from build123d import *

# Parameters (mm, degrees)
CROQUIS1_R              = 7.5
SALIENTE_EXTRUIR1_DEPTH = 10


with BuildPart() as part:
    # Croquis1 → Saliente-Extruir1 (new body)
    with BuildSketch(Plane(origin=(0, 0, 0), x_dir=(1, 0, 0), z_dir=(0, 1, 0))):
        with BuildLine():
            Line((-35, 35), (35, 35))
            Line((35, 35), (35, -25))
            ThreePointArc((35, -25), (32.071067812, -32.071067812), (25, -35))
            Line((25, -35), (-25, -35))
            ThreePointArc((-25, -35), (-32.071067812, -32.071067812), (-35, -25))
            Line((-35, -25), (-35, 35))
        make_face()
        Circle(CROQUIS1_R, mode=Mode.SUBTRACT)
    extrude(amount=SALIENTE_EXTRUIR1_DEPTH)


solid = part.part
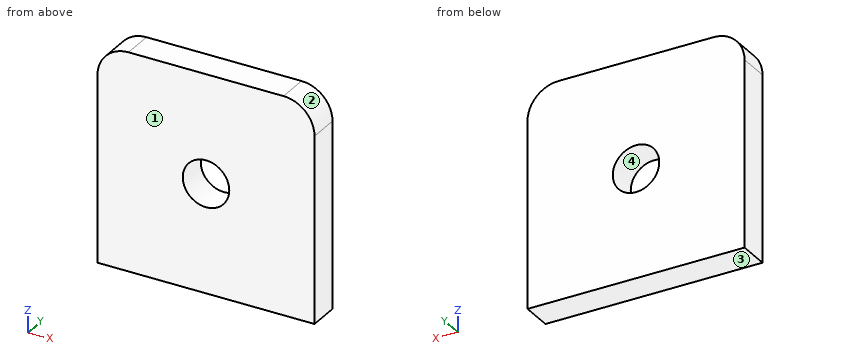
Read the model definition and answer for the solid it produces. Units are mm, in the model's axes. Face numbers are marked on the shaded views. Coordinates: 2 decimals unless noted, no trailing zeros. Write each loop counter-clockwise with the first axis right and the second up, starting at its lowest first coordinate (ties: lowest second). Pieces come first, ordered by that corner, then holes. Notation, with made-up numbers: (88.25, 7.5) -> (129.25, 7.5) arc R18 cw to (129.25, 21.5) -> close; hole circle Ø9 at (-9.5, 24). An arc over 180 degrees is marked (long way). Return JSON: item names as keys, results as strings.
(1) The part is cut by section B-B on y = 6.5. Give the vertices of the cut face in (x, z), then the cut area to 3 significant figures.
Answers below:
{"outline": "(-35, -35) -> (35, -35) -> (35, 25) arc R10 ccw to (25, 35) -> (-25, 35) arc R10 ccw to (-35, 25) -> close; hole circle Ø15 at (0, 0)", "area": "4,680 mm^2"}
(2) Each of these flat-tipped pins is pushed along its axis until it touches: P1, Ø6, axis at x = 20, z = -16.5, coming from the -Y side; P2, Ø3, axis at x = -27.5, y = 5, coming from the +Z side. Where does it stop, or does it pass through?
Answers below:
{"P1": "y = 0", "P2": "z = 34.95"}
(3) The part is cut by section C-C on z = 0. Give the vertices of the cut face in (x, y), then the cut area to 3 significant figures.
Answers below:
{"outline": "(-35, 0) -> (-7.5, 0) -> (-7.5, 10) -> (-35, 10) -> close; (7.5, 0) -> (35, 0) -> (35, 10) -> (7.5, 10) -> close", "area": "550 mm^2"}
(4) Consider line 1 along X through (y, z) = (6.25, 0); line 2 along X through (y, z) = (5.75, -6). Determine where each line is inside the solid, lowest interval first. Write a range as from..to.
Answers below:
{"line 1": "-35..-7.5, 7.5..35", "line 2": "-35..-4.5, 4.5..35"}
(5) The part is cut by section A-A on x = 0. Give the vertices of the cut face in (y, z), then the cut area to 3 significant figures.
Answers below:
{"outline": "(0, -35) -> (10, -35) -> (10, -7.5) -> (0, -7.5) -> close; (0, 7.5) -> (10, 7.5) -> (10, 35) -> (0, 35) -> close", "area": "550 mm^2"}
(6) For a pull along Z with two mould halves and no side action, classify the marked faces 1, 2, 3 and 4 as pulls with the +Z half, pulls with the -Z half, needs draft (parallel to the pull), parting line crosses it, or undercut.
Answers below:
{"face 1": "needs draft", "face 2": "pulls with the +Z half", "face 3": "pulls with the -Z half", "face 4": "undercut"}
